The listing builds one solid part. Answer for the finished solid, in the listing's coordinates (mm). A direction names the side the tool comes from. Give positions to 0.01 mm unless a question says otherwise; leave off trailing zeros. Write each loop counter-clockwise with the first axis right and the second up, starting at its lowest first coordinate (ties: lowest second). Pieces come first, ordered by that corner, then holes. Notation, with made-up numbers: (88, -27) -> (121, -27) arc R34 ccw to (121, 5) -> close; hole circle Ø5 at (-31.5, 25.5). An arc over 180 degrees is marked (long way). One line per question, with ' | ' between items.
from build123d import *

# Parameters (mm, degrees)
CROQUIS1_W              = 30
CROQUIS1_H              = 10
CROQUIS1_R              = 1.6
SALIENTE_EXTRUIR1_DEPTH = 5
CROQUIS2_R              = 2.8
CORTAR_EXTRUIR1_DEPTH   = 3
SALIENTE_EXTRUIR5_DEPTH = 10
SALIENTE_EXTRUIR6_DEPTH = 30
SALIENTE_EXTRUIR7_DEPTH = 10
REDONDEO1_R             = 5
REDONDEO2_R             = 5
SALIENTE_EXTRUIR8_DEPTH = 50


# Some blends are built 0.0001 mm under size
with BuildPart() as part:
    # Croquis1 → Saliente-Extruir1 (new body)
    with BuildSketch(Plane(origin=(0, 0, 0), x_dir=(1, 0, 0), z_dir=(0, 1, 0))):
        with Locations((15, 5)):
            Rectangle(CROQUIS1_W, CROQUIS1_H)
        with Locations(Location((5, 5, 0), (0, 0, 270))):
            Circle(CROQUIS1_R, mode=Mode.SUBTRACT)
        with Locations(Location((25, 5, 0), (0, 0, 270))):
            Circle(CROQUIS1_R, mode=Mode.SUBTRACT)
    extrude(amount=SALIENTE_EXTRUIR1_DEPTH)

    # Croquis2 → Cortar-Extruir1 (cut)
    with BuildSketch(Plane(origin=(0, 5, 0), x_dir=(1, 0, 0), z_dir=(0, 1, 0))):
        with Locations(Location((5, 5, 0), (0, 0, 270))):
            Circle(CROQUIS2_R)
        with Locations(Location((25, 5, 0), (0, 0, 270))):
            Circle(CROQUIS2_R)
    extrude(amount=-CORTAR_EXTRUIR1_DEPTH, mode=Mode.SUBTRACT)

    # Croquis6 → Saliente-Extruir5 (add)
    with BuildSketch(Plane.ZY):
        Polygon((-15, 16.781992624), (-10, 20.977490779), (-10, 16.781992624), (-10, 5), (0, 5), (0, 0), (-10, 0), (-15, 0), (-15, 12.586494468), (-20, 12.586494468), align=None)
    extrude(amount=SALIENTE_EXTRUIR5_DEPTH)

    # Croquis7 → Saliente-Extruir6 (add)
    with BuildSketch(Plane(origin=(0, 0, 0), x_dir=(0, 0, -1), z_dir=(1, 0, 0))):
        Polygon((10, 20.977490779), (10, 5), (10, 0), (15, 0), (15, 12.586494468), (20, 12.586494468), align=None)
    extrude(amount=SALIENTE_EXTRUIR6_DEPTH)

    # Croquis8 → Saliente-Extruir7 (add)
    with BuildSketch(Plane(origin=(30, 0, 0), x_dir=(0, 0, -1), z_dir=(1, 0, 0))):
        Polygon((0, 0), (15, 0), (15, 12.586494468), (20, 12.586494468), (10, 20.977490779), (10, 5), (0, 5), align=None)
    extrude(amount=SALIENTE_EXTRUIR7_DEPTH)

    # Redondeo1
    # the kernel refuses this fillet: 5 mm, written as the material it adds along each edge
    with BuildSketch(Plane(origin=(40, 5, -10), x_dir=(0, 1, 0), z_dir=(-1, 0, 0))) as redondeo1_piece_1_section:
        with BuildLine():
            CenterArc((REDONDEO1_R, -REDONDEO1_R), REDONDEO1_R, 90, 90)
            Line((0, -REDONDEO1_R), (0, 0))
            Line((0, 0), (REDONDEO1_R, 0))
        make_face()
    redondeo1_piece_1 = extrude(amount=50, mode=Mode.PRIVATE)
    redondeo1_piece_1 = redondeo1_piece_1 - Plane(origin=(5, 6.156265405, -5), x_dir=(0, 0, 1), z_dir=(0, 1, 0)) * Cylinder(2.8, 120, mode=Mode.PRIVATE)
    redondeo1_piece_1 = redondeo1_piece_1 - Plane(origin=(25, 6.156265405, -5), x_dir=(0, 0, 1), z_dir=(0, 1, 0)) * Cylinder(2.8, 120, mode=Mode.PRIVATE)
    add(redondeo1_piece_1)

    # Redondeo2
    redondeo2_edges = [part.edges().sort_by_distance(p)[0] for p in [
        (15, 12.586494468, -15),
    ]]
    fillet(redondeo2_edges, radius=REDONDEO2_R - 0.0001)  # a hair under: the kernel refuses the full size

    # Croquis9 → Saliente-Extruir8 (add)
    with BuildSketch(Plane.ZY.offset(10)):
        Polygon((-20, 12.586494468), (-25.717162805, 7.789225266), (-23.788799976, 5.491091937), (-10, 17.061268911), (-10, 20.977490779), align=None)
    extrude(amount=-SALIENTE_EXTRUIR8_DEPTH)


solid = part.part
Item 1: Find section B-B (y = 3). Write down the section's boundary in (x, z), then the cut area to 3 significant figures.
Answers below:
outline: (-10, -15) -> (40, -15) -> (40, 0) -> (-10, 0) -> close; hole circle Ø5.6 at (5, -5); hole circle Ø5.6 at (25, -5) | area: 701 mm²
Item 2: Determine the mould class of faces 1 (the face through (15, 4, -15)), 2 (the face through (5, 2, -3)), 3 (the face through (5.1, 3.5, -7.8)), 4 (the face through (40, 8, -13)) for opening direction X: pulls with the +X half, pulls with the -X half, needs draft (parallel to the pull), parting line crosses it, or undercut.
Answers below:
face 1: needs draft | face 2: undercut | face 3: undercut | face 4: pulls with the +X half
Item 3: Find section A-A (x = 5). Write down the section's boundary in (y, z), then the cut area to 3 significant figures.
Answers below:
outline: (0, -15) -> (7.59, -15) arc R5 cw to (11.39, -16.76) -> (5.49, -23.79) -> (7.79, -25.72) -> (20.98, -10) -> (10, -10) arc R5 cw to (5.86, -7.8) -> (2, -7.8) -> (2, -6.6) -> (0, -6.6) -> close; (0, -3.4) -> (2, -3.4) -> (2, -2.2) -> (5, -2.2) -> (5, 0) -> (0, 0) -> close | area: 167 mm²
Item 4: Find section D-D (y = 19). Write down the section's boundary in (x, z), then the cut area to 3 significant figures.
Answers below:
outline: (-10, -12.36) -> (40, -12.36) -> (40, -10) -> (-10, -10) -> close | area: 118 mm²
Item 5: Consider line 1 (X direction, y = 1.25, z = -5); line 2 (X direction, y = 3.7, z = -5); line 3 (Z direction, x = 25, y = 4.5). Determine where each line is inside the solid, lowest interval first. Write a range as [from, to].
Answers below:
line 1: [-10, 3.4], [6.6, 23.4], [26.6, 40] | line 2: [-10, 2.2], [7.8, 22.2], [27.8, 40] | line 3: [-15, -7.8], [-2.2, 0]
Item 6: Find section C-C (x = -5). Write down the section's boundary in (y, z).
Answers below:
outline: (0, -15) -> (7.59, -15) arc R5 cw to (11.39, -16.76) -> (5.49, -23.79) -> (7.79, -25.72) -> (20.98, -10) -> (10, -10) arc R5 cw to (5, -5) -> (5, 0) -> (0, 0) -> close
Item 7: Flat-ended cylindrical pins translate along their axes: pin 1 (9 mm diameter, centred on x = 23, y = 14.5, fed in from +Z); pin 2 (10 mm diameter, centred on x = 14.5, y = 2.5, fed in from -Z); pin 3 (3 mm diameter, centred on x = -1, y = 11, fed in from -Z). Find the tip coordinate at first contact, or state that the pin passes through.
Answers below:
pin 1: z = -10 | pin 2: z = -25.47 | pin 3: z = -23.68
Item 8: A tool of negligible diameter and unlimited length cuts with its end or side. For faces 5 (the face through (15, 16, -10)), 6 (the face through (-10, 8, -13)), 7 (the face through (25, 2, -3)), 8 (the face through (24.03, 0.99, -6.27)), 9 (the face through (15.35, 9.655, -15.448)), from which of +Z, -Z, +X, -X, +Y, -Y can it reach the whole face along a straight path? Write none if from no direction.
Answers below:
face 5: +Z, +X, -X, +Y | face 6: +Z, -Z, -X, +Y, -Y | face 7: +Y | face 8: +Y, -Y | face 9: +X, -X, -Y
